The listing builds one solid part. Answer for the finished solid, in the listing's coordinates (mm). Round coordinates to 2 decimals unless told otherwise and drop trailing zeros. Loops run counter-clockwise (first coordinate to the right, second up) from the corner with the lowest first, then second, coordinate; pieces in that order, holes last. Notation, with made-up numbers: (72, 14.5) -> (88, 14.5) arc R14 ccw to (88, 32.5) -> close; hole circle Ø8 at (-34.5, 54.25). An arc over 180 degrees is marked (long way). Use a Markdown table: item, result. Add a question column.
Q1. Given pin 1 Ø1.5 at (y, z) = (74, 1) entering from -X; pin 2 Ø0.9 at (x, z) = (136.5, 1.5) entering from +Y; pin 3 Ø1.5 at (y, z) = (113, 1.5) entering from +X, each flat-ended and moving along its own axis, determine where each tip first touches the part or whether it passes through.
Q2. Section A-A on y = 147.5 is taken. Give the vertices of the cut face in (x, z), then the cut area to 3 significant figures.
Q3. Section B-B on y = 113 is taken. Give the vertices of the cut face in (x, z), then the cut area to 3 significant figures.
Q4. Section C-C on x = 128 is taken. Give the vertices of the cut face in (y, z).
Q5. Consider line 1 (X direction, y = 19.5, z = 0.9); line 2 (X direction, y = 132.5, z = 1.2); line 3 (Y direction, x = 68.5, z = 1.2). Determine where each line is inside the solid, lowest interval first.
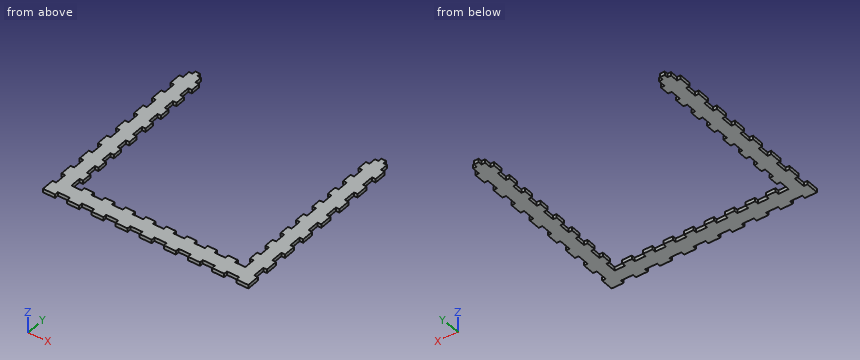
from build123d import *

# Parameters (mm, degrees)
F1_DEPTH = 3


with BuildPart() as f1:
    # F0 (on Top) → F1 (new body)
    with BuildSketch(Plane.XY):
        Polygon((0, 10.5), (0, 0), (10, 0), (10, 3), (20, 3), (20, 0), (30, 0), (30, 3), (40, 3), (40, 0), (50, 0), (50, 3), (60, 3), (60, 0), (70, 0), (70, 3), (80, 3), (80, 0), (90, 0), (90, 3), (100, 3), (100, 0), (110, 0), (110, 3), (120, 3), (120, 0), (130, 0), (130, 3), (140, 3), (140, 0), (150, 0), (150, 3), (160, 3), (160, 0), (170, 0), (170, 10.5), (167, 10.5), (167, 20.5), (170, 20.5), (170, 30.5), (167, 30.5), (167, 40.5), (170, 40.5), (170, 50.5), (167, 50.5), (167, 60.5), (170, 60.5), (170, 70.5), (167, 70.5), (167, 80.5), (170, 80.5), (170, 90.5), (167, 90.5), (167, 100.5), (170, 100.5), (170, 110.5), (167, 110.5), (167, 120.5), (170, 120.5), (170, 130.5), (167, 130.5), (167, 140.5), (170, 140.5), (170, 150.5), (167, 150.5), (167, 157), (164, 157), (164, 160), (160, 160), (160, 157), (157, 157), (157, 151), (154, 151), (154, 143), (157, 143), (157, 134), (154, 134), (154, 126), (157, 126), (157, 117), (154, 117), (154, 109), (157, 109), (157, 100), (154, 100), (154, 92), (157, 92), (157, 82), (154, 82), (154, 74), (157, 74), (157, 65), (154, 65), (154, 57), (157, 57), (157, 48), (154, 48), (154, 40), (157, 40), (157, 31), (154, 31), (154, 23), (157, 23), (157, 14), (148.5, 14), (148.5, 17), (140.5, 17), (140.5, 14), (131.5, 14), (131.5, 17), (123.5, 17), (123.5, 14), (114.5, 14), (114.5, 17), (106.5, 17), (106.5, 14), (97.5, 14), (97.5, 17), (89.5, 17), (89.5, 14), (80.5, 14), (80.5, 17), (72.5, 17), (72.5, 14), (63.5, 14), (63.5, 17), (55.5, 17), (55.5, 14), (46.5, 14), (46.5, 17), (38.5, 17), (38.5, 14), (29.5, 14), (29.5, 17), (21.5, 17), (21.5, 14), (13, 14), (13, 23), (16, 23), (16, 31), (13, 31), (13, 40), (16, 40), (16, 48), (13, 48), (13, 57), (16, 57), (16, 65), (13, 65), (13, 74), (16, 74), (16, 82), (13, 82), (13, 92), (16, 92), (16, 100), (13, 100), (13, 109), (16, 109), (16, 117), (13, 117), (13, 126), (16, 126), (16, 134), (13, 134), (13, 143), (16, 143), (16, 151), (13, 151), (13, 157), (10, 157), (10, 160), (6, 160), (6, 157), (3, 157), (3, 150.5), (0, 150.5), (0, 140.5), (3, 140.5), (3, 130.5), (0, 130.5), (0, 120.5), (3, 120.5), (3, 110.5), (0, 110.5), (0, 100.5), (3, 100.5), (3, 90.5), (0, 90.5), (0, 80.5), (3, 80.5), (3, 70.5), (0, 70.5), (0, 60.5), (3, 60.5), (3, 50.5), (0, 50.5), (0, 40.5), (3, 40.5), (3, 30.5), (0, 30.5), (0, 20.5), (3, 20.5), (3, 10.5), align=None)
    extrude(amount=F1_DEPTH)


solid = f1.part
Checked values:
| question | item | result |
|---|---|---|
| 1 | pin 1 | stops at x = 3 |
| 1 | pin 2 | stops at y = 14 |
| 1 | pin 3 | stops at x = 167 |
| 2 | outline | (0, 0) -> (16, 0) -> (16, 3) -> (0, 3) -> close; (154, 0) -> (170, 0) -> (170, 3) -> (154, 3) -> close |
| 2 | area | 96.0 mm2 |
| 3 | outline | (3, 0) -> (16, 0) -> (16, 3) -> (3, 3) -> close; (154, 0) -> (167, 0) -> (167, 3) -> (154, 3) -> close |
| 3 | area | 78.0 mm2 |
| 4 | outline | (0, 0) -> (17, 0) -> (17, 3) -> (0, 3) -> close |
| 5 | line 1 | x = 3 to 13, 157 to 167 |
| 5 | line 2 | x = 3 to 16, 154 to 167 |
| 5 | line 3 | y = 0 to 14 |
